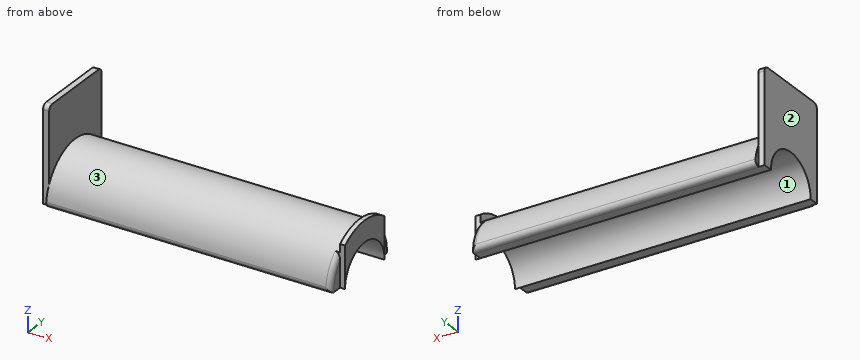
from build123d import *

# Parameters (mm, degrees)
F1_DEPTH     = 115
F3_DEPTH     = 2
F5_DEPTH     = 2.5
F6_R         = 2
F8_DEPTH     = 5
F10_DEPTH    = 119.5
F11_T1_DEPTH = 126.2328463215
F11_T6_ANGLE = 78.4675131369
F12_T1_DEPTH = 124.2328463215
F12_T6_ANGLE = 71.5045093033


# Not quite as in the source:
# - a fillet or chamfer that OpenCascade refuses, or shapes differently, is made with other operations: its cross-section is extruded or revolved along the edge and cut away or added


with BuildPart() as f1:
    # F0 (on Right) → F1 (new body)
    with BuildSketch(Plane.YZ):
        with BuildLine():
            Line((-18.5, 0), (18.5, 0))
            ThreePointArc((18.5, 0), (0, 18.5), (-18.5, 0))
        make_face()
    extrude(amount=-F1_DEPTH)

    # F2 (on face) → F3 (join)
    with BuildSketch(Plane.YZ):
        with BuildLine():
            Line((12.5, 21), (-12.5, 21))
            Line((-12.5, 21), (-12.5, 13.638181697))
            ThreePointArc((-12.5, 13.638181697), (0, 18.5), (12.5, 13.638181697))
            Line((12.5, 13.638181697), (12.5, 21))
        make_face()
        with BuildLine():
            ThreePointArc((12.5, 13.638181697), (0, 18.5), (-12.5, 13.638181697))
            Line((-12.5, 13.638181697), (-12.5, 0))
            Line((-12.5, 0), (12.5, 0))
            Line((12.5, 0), (12.5, 13.638181697))
        make_face()
    extrude(amount=F3_DEPTH)

    # F4 (on face) → F5 (join)
    with BuildSketch(Plane(origin=(-115, 0, 0), x_dir=(0, -1, 0), z_dir=(-1, 0, 0))):
        with BuildLine():
            Line((-16.5, 8.3666002653), (-16.5, 0))
            Line((-16.5, 0), (16.5, 0))
            Line((16.5, 0), (16.5, 8.3666002653))
            ThreePointArc((16.5, 8.3666002653), (0, 18.5), (-16.5, 8.3666002653))
        make_face()
        with BuildLine():
            Line((-16.5, 38.5), (-16.5, 8.3666002653))
            ThreePointArc((-16.5, 8.3666002653), (0, 18.5), (16.5, 8.3666002653))
            Line((16.5, 8.3666002653), (16.5, 38.5))
            Line((16.5, 38.5), (-16.5, 38.5))
        make_face()
    extrude(amount=F5_DEPTH)

    # F6
    f6_edges = [f1.edges().sort_by_distance(p)[0] for p in [
        (-116.25, 16.5, 38.5),
        (-116.25, -16.5, 38.5),
    ]]
    fillet(f6_edges, radius=F6_R)

    # F7 (on face) → F8 (cut)
    with BuildSketch(Plane.YZ.offset(2)):
        with BuildLine():
            Line((-12.5, 21), (-12.5, 16.8745370307))
            ThreePointArc((-12.5, 16.8745370307), (-6.5815925928, 19.9419818208), (1.93e-08, 21))
            Line((1.93e-08, 21), (-12.5, 21))
        make_face()
        with BuildLine():
            ThreePointArc((1.93e-08, 21), (6.5815926111, 19.9419818148), (12.5, 16.8745370307))
            Line((12.5, 16.8745370307), (12.5, 21))
            Line((12.5, 21), (1.93e-08, 21))
        make_face()
    extrude(amount=-F8_DEPTH, mode=Mode.SUBTRACT)

    # F9 (on face) → F10 (cut, through all)
    with BuildSketch(Plane.YZ.offset(2)):
        with BuildLine():
            Line((-12.5, 0), (12.5, 0))
            ThreePointArc((12.5, 0), (0, 12.5), (-12.5, 0))
        make_face()
    extrude(amount=-F10_DEPTH, mode=Mode.SUBTRACT)

    # F11: fillet of radius 2 on 2 edges, made by hand

    # F11_s2 → F11_t1 (cut)
    with BuildSketch(Plane.YZ.offset(-120.6164231607)):
        with BuildLine():
            ThreePointArc((18.3635926092, 2.2424242424), (17.8758119724, 0.6742640694), (16.3783393542, 0))
            Line((16.3783393542, 0), (18.5, 0))
            ThreePointArc((18.5, 0), (18.4658666635, 1.1232846321), (18.3635926092, 2.2424242424))
        make_face()
    extrude(amount=F11_T1_DEPTH, mode=Mode.SUBTRACT)


with BuildPart() as f11_tool4:
    # F11_s5 → F11_t6 (revolve)
    with BuildSketch(Plane(origin=(0, 0, 0), x_dir=(1, 0, 0), z_dir=(0, 0.8908514497, 0.454294722))):
        with BuildLine():
            ThreePointArc((-2, -18.5), (-0.5857864376, -17.9142135624), (0, -16.5))
            Line((0, -16.5), (0, -18.5))
            Line((0, -18.5), (-2, -18.5))
        make_face()
    revolve(axis=Axis((0, 0, 0), (1, 0, 0)), revolution_arc=F11_T6_ANGLE)

    split(bisect_by=Plane.XZ.offset(12.5), keep=Keep.TOP)


with BuildPart() as f1_1:
    add(f1.part)

    # F11_t3: cut F11_tool4
    add(f11_tool4.part, mode=Mode.SUBTRACT)

    # F12: fillet of radius 2 on 2 edges, made by hand

    # F12_s2 → F12_t1 (cut)
    with BuildSketch(Plane.YZ.offset(-120.6164231607)):
        with BuildLine():
            ThreePointArc((-18.3635926092, 2.2424242424), (-17.8758119724, 0.6742640694), (-16.3783393542, 0))
            Line((-16.3783393542, 0), (-18.5, 0))
            ThreePointArc((-18.5, 0), (-18.4658666635, 1.1232846321), (-18.3635926092, 2.2424242424))
        make_face()
    extrude(amount=F12_T1_DEPTH, mode=Mode.SUBTRACT)


with BuildPart() as f12_tool4:
    # F12_s5 → F12_t6 (revolve)
    with BuildSketch(Plane(origin=(0, 0, 0), x_dir=(1, 0, 0), z_dir=(0, -0.1482330737, -0.9889524538))):
        with BuildLine():
            ThreePointArc((-2, -18.5), (-0.5857864376, -17.9142135624), (0, -16.5))
            Line((0, -16.5), (0, -18.5))
            Line((0, -18.5), (-2, -18.5))
        make_face()
    revolve(axis=Axis((0, 0, 0), (1, 0, 0)), revolution_arc=F12_T6_ANGLE)

    split(bisect_by=Plane.XZ.offset(-12.5), keep=Keep.BOTTOM)


with BuildPart() as f1_2:
    add(f1_1.part)

    # F12_t3: cut F12_tool4
    add(f12_tool4.part, mode=Mode.SUBTRACT)


solid = f1_2.part
The model under review builds one solid part; all positions refer to its coordinate system, in mm. Face numbers are marked on the shaded views. Round coordinates to 2 decimals unless told otherwise and drop trailing zeros. Loops run counter-clockwise (first coordinate to the right, second up) from the corner with the lowest first, then second, coordinate; pieces in that order, holes last. Notation, with made-up numbers: (-12.75, -6) -> (-3.75, -6) arc R21 cw to (-3.75, 13) -> close; hole circle Ø10 at (42.5, -6.5). An arc over 180 degrees is marked (long way). Write item = value, one per line. Start each with the question number.
Item 1: Take a section at D-D on z = 32.5. Give the boundary of the cut face in (x, y), plus the area to 3 significant figures.
Item 2: Take a section at B-B on z = 15. Give the boundary of the cut face in (x, y), plus the area to 3 significant figures.
Item 3: Mouldability with a two-part tool opening along Y and no side actions: class the marked faces 1, 2 and 3 as released by +Y, released by -Y, zero draft, split by the parting line, or undercut.
Item 4: Take a section at A-A on x = -55.5. Give the boundary of the cut face in (y, z).
Item 5: To check wall thickness, follow L1, parallel to X at y = 4.5, z = 19; L2, parallel to X at y = -13.5, z = 28; L3, parallel to Y at x = -23.5, z = 3. State the ranges of each line that lie inside material, in increasing order.
Item 6: Insertion check: pin 1 (1 mm diameter, centred on x = -34, z = 8, fed in from -Y); pin 2 (1.5 mm diameter, centred on y = 17.5, z = 5.5, fed in from -X); pin 3 (5 mm diameter, centred on x = -11, y = 6, fed in from -Z); pin 4 (4.5 mm diameter, centred on y = 14, z = 4, fed in from +X). Each pin has a flat end and moves straight along its axis. Give the tip position at first contact, or say it passes through.
Item 7: Take a section at C-C on y = 6. Give the boundary of the cut face in (x, z).
Result:
q1.outline = (-117.5, -16.5) -> (-115, -16.5) -> (-115, 16.5) -> (-117.5, 16.5) -> close
q1.area = 82.5 mm²
q2.outline = (-117.5, -16.5) -> (-115, -16.5) -> (-115, -10.83) -> (0, -10.83) -> (0, -12.5) -> (2, -12.5) -> (2, 12.5) -> (0, 12.5) -> (0, 10.83) -> (-115, 10.83) -> (-115, 16.5) -> (-117.5, 16.5) -> close
q2.area = 2,620 mm²
q3.face_1 = undercut
q3.face_2 = zero draft
q3.face_3 = split by the parting line
q4.outline = (-18.36, 2.24) arc R2 ccw to (-16.38, 0) -> (-12.5, 0) arc R12.5 cw to (12.5, 0) -> (16.38, 0) arc R2 ccw to (18.36, 2.24) arc R18.5 ccw to start
q5.L1 = -117.5 to -115, 0 to 2
q5.L2 = -117.5 to -115
q5.L3 = -18.26 to -12.13, 12.13 to 18.26
q6.pin_1 = -16.91
q6.pin_2 = -115
q6.pin_3 = 9.17
q6.pin_4 = 2
q7.outline = (-117.5, 10.97) -> (2, 10.97) -> (2, 20.12) -> (0, 20.12) -> (0, 17.5) -> (-115, 17.5) -> (-115, 38.5) -> (-117.5, 38.5) -> close
